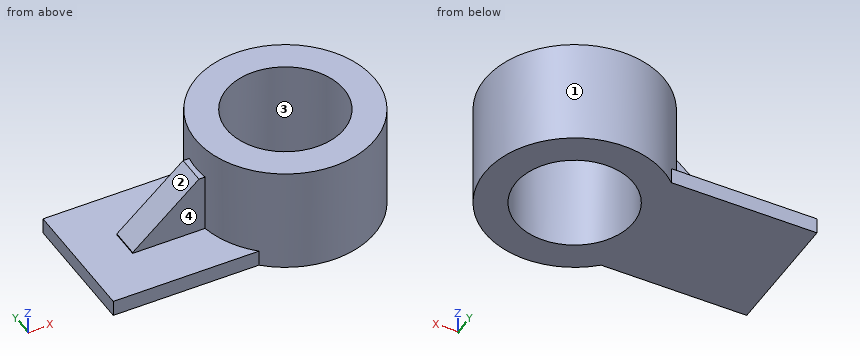
```python
from build123d import *

# Parameters (mm, degrees)
F0_R          = 42.6730408219
F0_R_2        = 28.0004794719
F1_DEPTH      = 50.8
F2_W          = 70.7396827638
F2_H          = 61.8972182274
F3_DEPTH      = 7.62
F4_W          = 47.3499465734
F4_H          = 13.9767918736
F5_DEPTH      = 27.94
F7_DEPTH      = 25.4
F7_DEPTH_BACK = 25.4


with BuildPart() as f1:
    # F0 (on Top) → F1 (new body)
    with BuildSketch(Plane.XY):
        with Locations((42.7860990167, 0)):
            Circle(F0_R)
        with Locations((42.7860990167, 0)):
            Circle(F0_R_2, mode=Mode.SUBTRACT)
    extrude(amount=F1_DEPTH)

    # F2 (on Top) → F3 (join)
    with BuildSketch(Plane.XY):
        with Locations((-20.7568462938, 0)):
            Rectangle(F2_W, F2_H)
    extrude(amount=F3_DEPTH)

    # F4 (on face) → F5 (join)
    with BuildSketch(Plane.XY.offset(7.62)):
        with Locations((-10.2029433474, 0)):
            Rectangle(F4_W, F4_H)
    extrude(amount=F5_DEPTH)

    # F6 (on Front) → F7 (cut, two sides)
    with BuildSketch(Plane.XZ) as f7_sk:
        Polygon((-34.1631546617, 37.5091433525), (-34.1631546617, 7.8441174701), (0, 37.5091433525), align=None)
    extrude(amount=-F7_DEPTH, mode=Mode.SUBTRACT)
    extrude(f7_sk.sketch, amount=F7_DEPTH_BACK, mode=Mode.SUBTRACT)


solid = f1.part
```
Can you work these out from the model? Positions are in its coordinate system, mm. Face numbers are marked on the shaded views. Give positions to 0.01 mm unless a question says otherwise; leave off trailing zeros. Order: outer loops, then holes, each group sorted by start corner. A loop starts at its lowest first (then second) coordinate and runs counter-clockwise, first axis right, second up. Notation, with made-up numbers: (58, 23) - (68, 23) arc R23 cw to (68, 43) - close; hole circle Ø11 at (61, 34.5). An arc over 180 degrees is marked (long way). Use a Markdown table: item, result. Add a question column.
Q1. I'm going to push flat-ended pins straight in: pin 1 (1.5 mm diameter, centred on y = 32.5, z = 34.5, fed in from +X); pin 2 (4 mm diameter, centred on x = -22, z = 2.5, fed in from -Y); pin 3 (8 mm diameter, centred on x = -26, z = 13, fed in from +Y). Where does each tip first touch, or does it pass through?
Q2. If we section it at A-A on y = 0: Write out the boundary of the cut face in (x, z), plus the area to 3 significant figures.
Q3. If we section it at C-C on z = 18.5: Write out the boundary of the cut face in (x, y), plus the area to 3 significant figures.
Q4. If we section it at D-D on y = -26: Write out the boundary of the cut face in (x, z), plus the area to 3 significant figures.
Q5. If we section it at B-B on x = 31: Write out the boundary of the cut face in (y, z), plus the area to 3 significant figures.
Q6. If we mould it in two halves opening along X, with no side actions, what happens to the marked faces 1, 2, 3 and 4? For each: released by +X, released by -X, zero draft, split by the parting line, or undercut.
Q7. Please list where these lines run through material, in increasing order: line 1 along Z through (x, y) = (-23, -12.5); line 2 along Y through (x, z) = (36, 12); line 3 along X through (y, z) = (-10, 20).
Answers follow:
| question | item | result |
|---|---|---|
| 1 | pin 1 | stops at x = 71.3 |
| 1 | pin 2 | stops at y = -30.95 |
| 1 | pin 3 | stops at y = 6.99 |
| 2 | outline | (-56.13, 0) - (14.79, 0) - (14.79, 50.8) - (0.11, 50.8) - (0.11, 35.56) - (-2.24, 35.56) - (-33.88, 8.09) - (-33.88, 7.62) - (-56.13, 7.62) - close; (70.79, 0) - (85.46, 0) - (85.46, 50.8) - (70.79, 50.8) - close |
| 2 | area | 2,430 mm^2 |
| 3 | outline | (-21.89, -6.99) - (0.69, -6.99) arc R42.67 ccw (long way) to (0.69, 6.99) - (-21.89, 6.99) - close; hole circle Ø56 at (42.79, 0) |
| 3 | area | 3,570 mm^2 |
| 4 | outline | (-56.13, 0) - (32.39, 0) - (32.39, 50.8) - (8.95, 50.8) - (8.95, 7.62) - (-56.13, 7.62) - close; (53.18, 0) - (76.62, 0) - (76.62, 50.8) - (53.18, 50.8) - close |
| 4 | area | 2,880 mm^2 |
| 5 | outline | (-41.01, 0) - (-25.4, 0) - (-25.4, 50.8) - (-41.01, 50.8) - close; (25.4, 0) - (41.01, 0) - (41.01, 50.8) - (25.4, 50.8) - close |
| 5 | area | 1,590 mm^2 |
| 6 | face 1 | split by the parting line |
| 6 | face 2 | released by -X |
| 6 | face 3 | undercut |
| 6 | face 4 | zero draft |
| 7 | line 1 | z = 0 to 7.62 |
| 7 | line 2 | y = -42.13 to -27.17, 27.17 to 42.13 |
| 7 | line 3 | x = 1.3 to 16.63, 68.94 to 84.27 |
